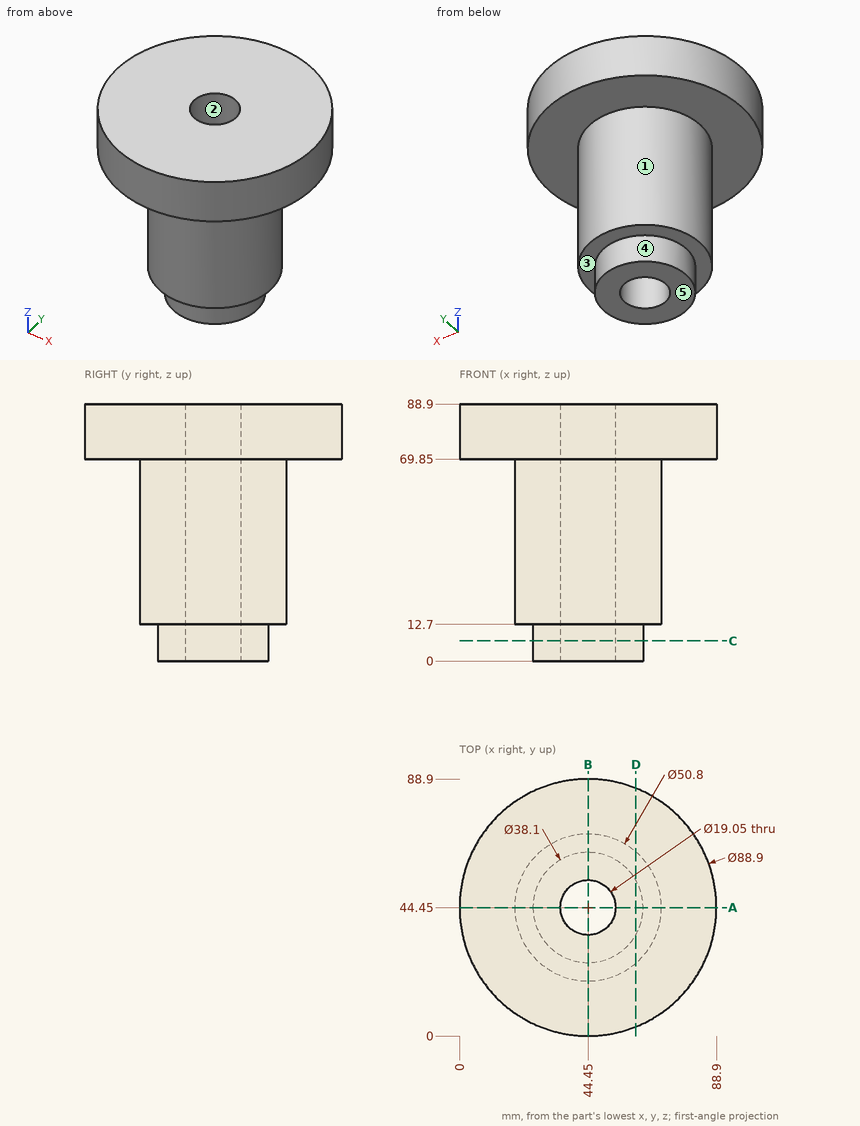
Check sheet for the drawn part. Datum: minimum x, y, z corner. Units: mm. A direction names the side the tool comes from. Round coordinates to 2 decimals unless told otherwise and drop trailing zeros. Loops run counter-clockwise (first coordinate to the right, second up) from the corner with the lowest first, then second, coordinate; pieces in that order, holes last. Notation, with made-up numbers: M 33,12.5 L 88,12.5 A29 ccw 88,44.5 Z; hole C -27.5,-21.75 d3. An arc over 180 degrees is marked long. Write each question's results on one line, items separated by ' | '.
1) Access from +Z, -Z, +X, -X, +Y, -Y to the whole of each face (thin tool, end or side, straight path). Record for the marked faces 4 and 5.
Checks:
face 4: -Z | face 5: -Z, +X, -X, +Y, -Y
2) Section check C-C on z = 7. Record the boundary of the cut face in (x, y) (3 decimals).
Checks:
outline: C 44.45,44.45 d38.1; hole C 44.45,44.45 d19.05
3) Scan lines: L1, parallel to Y at x = 44.45, z = 45 (3 decimals); L2, parallel to Z at x = 65.5, y = 61. Record each from-to range of solid material in increasing order. Write a range as from..to.
Checks:
L1: y = 19.05..34.925, 53.975..69.85 | L2: z = 69.85..88.9
4) Gauge pin test, flat ends, axial feed: P1, Ø12, axis at y = 38.5, z = 68.5, coming from the +X side; P2, Ø15, axis at x = 44.45, y = 44.45, coming from the +Z side; P3, Ø6, axis at x = 11, y = 23.5, coming from the -Z side; P4, Ø4, axis at y = 24.5, z = 58, coming from the +X side. Record the tip position at first contact, or that the pin passes through.
Checks:
P1: stops at x = 88.9 | P2: passes through | P3: stops at z = 69.85 | P4: stops at x = 62.42
5) Section check D-D on x = 61. Record the boundary of the cut face in (y, z).
Checks:
outline: M 3.2,69.85 L 25.18,69.85 L 25.18,12.7 L 35.02,12.7 L 35.02,0 L 53.88,0 L 53.88,12.7 L 63.72,12.7 L 63.72,69.85 L 85.7,69.85 L 85.7,88.9 L 3.2,88.9 Z
6) Section check A-A on y = 44.45. Record the boundary of the cut face in (x, z) (3 decimals), then the cut area to 3 significant figures.
Checks:
outline: M 0,69.85 L 19.05,69.85 L 19.05,12.7 L 25.4,12.7 L 25.4,0 L 34.925,0 L 34.925,88.9 L 0,88.9 Z; M 53.975,0 L 63.5,0 L 63.5,12.7 L 69.85,12.7 L 69.85,69.85 L 88.9,69.85 L 88.9,88.9 L 53.975,88.9 Z | area: 3,390 mm2
7) Mould release check, pull along Y, two halves, no side actions. Record for the marked faces 1, 2 and 3: released by +Y, released by -Y, zero draft, split by the parting line, or undercut.
Checks:
face 1: split by the parting line | face 2: undercut | face 3: zero draft
